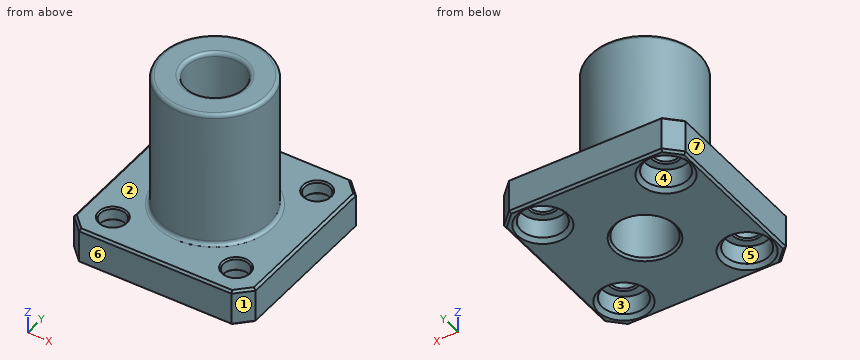
from build123d import *

# Parameters (mm, degrees)
SKETCH1_W                               = 25
SKETCH1_H                               = 25
SKETCH1_R                               = 4
BOSS_EXTRUDE1_DEPTH                     = 5
SKETCH2_R                               = 7.5
SKETCH2_R_2                             = 4
BOSS_EXTRUDE2_DEPTH                     = 19
CHAMFER1_SIZE                           = 2
CBORE_FOR_M3_PAN_HEAD_SCREW1_AT_2_COUNT = 2
CBORE_FOR_M3_PAN_HEAD_SCREW1_AT_2_PITCH = 16.970562748
CBORE_FOR_M3_PAN_HEAD_SCREW1_AT_3_COUNT = 2
CBORE_FOR_M3_PAN_HEAD_SCREW1_AT_3_PITCH = 24
CBORE_FOR_M3_PAN_HEAD_SCREW1_AT_4_COUNT = 2
CBORE_FOR_M3_PAN_HEAD_SCREW1_AT_4_PITCH = 16.970562748
CHAMFER2_SIZE                           = 0.3
FILLET1_R                               = 0.5
FILLET2_R                               = 0.5
CHAMFER3_SIZE                           = 0.3
FILLET3_R                               = 0.5
CHAMFER4_SIZE                           = 0.2


with BuildPart() as part:
    # Sketch1 → Boss-Extrude1 (new body)
    with BuildSketch(Plane.XY):
        Rectangle(SKETCH1_W, SKETCH1_H)
        Circle(SKETCH1_R, mode=Mode.SUBTRACT)
    extrude(amount=BOSS_EXTRUDE1_DEPTH)

    # Sketch2 → Boss-Extrude2 (add)
    with BuildSketch(Plane.XY.offset(5)):
        Circle(SKETCH2_R)
        Circle(SKETCH2_R_2, mode=Mode.SUBTRACT)
    extrude(amount=BOSS_EXTRUDE2_DEPTH)

    # Chamfer1
    chamfer1_edges = [part.edges().sort_by_distance(p)[0] for p in [
        (12.5, -12.5, 2.5),
        (-12.5, -12.5, 2.5),
        (-12.5, 12.5, 2.5),
        (12.5, 12.5, 2.5),
    ]]
    chamfer(chamfer1_edges, length=CHAMFER1_SIZE)

    # Sketch4 → CBORE for M3 Pan Head Screw1 (revolve, cut)
    with BuildSketch(Plane(origin=(8.485281374, 8.485281374, 0), x_dir=(0, 1, 0), z_dir=(1, 0, 0))):
        Polygon((0, 0), (0, 24), (1.75, 24), (1.75, 3.1), (3, 3.1), (3, 0.525), (3.525, 0), align=None)
    cbore_for_m3_pan_head_screw1 = revolve(axis=Axis((8.485281374, 8.485281374, -6.35), (0, 0, 1)), mode=Mode.SUBTRACT)

    # CBORE for M3 Pan Head Screw1 at 2: CBORE for M3 Pan Head Screw1 ×2
    with Locations(*[(-i * CBORE_FOR_M3_PAN_HEAD_SCREW1_AT_2_PITCH, 0, 0) for i in range(1, CBORE_FOR_M3_PAN_HEAD_SCREW1_AT_2_COUNT)]):
        add(cbore_for_m3_pan_head_screw1, mode=Mode.SUBTRACT)

    # CBORE for M3 Pan Head Screw1 at 3: CBORE for M3 Pan Head Screw1 ×2
    with Locations(*[Vector(-0.7071067811865676, -0.7071067811865276, 0) * (i * CBORE_FOR_M3_PAN_HEAD_SCREW1_AT_3_PITCH) for i in range(1, CBORE_FOR_M3_PAN_HEAD_SCREW1_AT_3_COUNT)]):
        add(cbore_for_m3_pan_head_screw1, mode=Mode.SUBTRACT)

    # CBORE for M3 Pan Head Screw1 at 4: CBORE for M3 Pan Head Screw1 ×2
    with Locations(*[(0, -i * CBORE_FOR_M3_PAN_HEAD_SCREW1_AT_4_PITCH, 0) for i in range(1, CBORE_FOR_M3_PAN_HEAD_SCREW1_AT_4_COUNT)]):
        add(cbore_for_m3_pan_head_screw1, mode=Mode.SUBTRACT)

    # Chamfer2
    chamfer2_edges = [part.edges().sort_by_distance(p)[0] for p in [
        (-12.5, 0, 0),
        (-12.5, 0, 5),
        (12.5, 0, 0),
        (0, -12.5, 0),
        (0, 12.5, 0),
        (11.5, 11.5, 0),
        (11.5, -11.5, 0),
        (-11.5, -11.5, 0),
        (-11.5, 11.5, 0),
        (0, 12.5, 5),
        (12.5, 0, 5),
        (0, -12.5, 5),
        (11.5, 11.5, 5),
        (11.5, -11.5, 5),
        (-11.5, -11.5, 5),
        (-11.5, 11.5, 5),
    ]]
    chamfer(chamfer2_edges, length=CHAMFER2_SIZE)

    # Fillet1
    fillet1_edges = [part.edges().sort_by_distance(p)[0] for p in [
        (-7.5, 0, 24),
    ]]
    fillet(fillet1_edges, radius=FILLET1_R)

    # Fillet2
    fillet2_edges = [part.edges().sort_by_distance(p)[0] for p in [
        (-4, 0, 24),
    ]]
    fillet(fillet2_edges, radius=FILLET2_R)

    # Chamfer3
    chamfer3_edges = [part.edges().sort_by_distance(p)[0] for p in [
        (-4, 0, 0),
    ]]
    chamfer(chamfer3_edges, length=CHAMFER3_SIZE)

    # Fillet3
    fillet3_edges = [part.edges().sort_by_distance(p)[0] for p in [
        (-7.5, 0, 5),
    ]]
    fillet(fillet3_edges, radius=FILLET3_R)

    # Chamfer4
    chamfer4_edges = [part.edges().sort_by_distance(p)[0] for p in [
        (8.485281374, -10.235281374, 5),
        (8.485281374, -10.235281374, 3.1),
        (-8.485281374, -10.235281374, 5),
        (-8.485281374, -10.235281374, 3.1),
        (-8.485281374, 6.735281374, 5),
        (-8.485281374, 6.735281374, 3.1),
        (8.485281374, 6.735281374, 5),
        (8.485281374, 6.735281374, 3.1),
    ]]
    chamfer(chamfer4_edges, length=CHAMFER4_SIZE)


solid = part.part
Part model, mm, in its own coordinate system. Face numbers are marked on the shaded views. A direction names the side the tool comes from. Coordinates: 2 decimals unless noted, no trailing zeros. Write each loop counter-clockwise with the first axis right and the second up, starting at its lowest first coordinate (ties: lowest second). Pieces come first, ordered by that corner, then holes. Notation, with made-up numbers: (8.5, 25) - (43.5, 25) arc R31 ccw to (43.5, 58) - close; hole circle Ø9 at (57.25, -24.75). An arc over 180 degrees is marked (long way). Put each result on its own line as item: value.
1. 3-axis set-ups, long thin cutter, end or side, ignore diameter. For the marked faces 1, 2 and 3: which of +Z, -Z, +X, -X, +Y, -Y reach the whole face in a straight line?
Final values:
face 1: +Z, -Z, +X, -Y
face 2: +Z
face 3: -Z
2. Band-saw the part on A-A (y = 0). Write the cut outline in (x, z).
Final values:
outline: (-12.5, 0.3) - (-12.2, 0) - (-4.3, 0) - (-4, 0.3) - (-4, 23.5) arc R0.5 ccw to (-4.5, 24) - (-7, 24) arc R0.5 ccw to (-7.5, 23.5) - (-7.5, 5.5) arc R0.5 cw to (-8, 5) - (-12.2, 5) - (-12.5, 4.7) - close; (4, 0.3) - (4.3, 0) - (12.2, 0) - (12.5, 0.3) - (12.5, 4.7) - (12.2, 5) - (8, 5) arc R0.5 cw to (7.5, 5.5) - (7.5, 23.5) arc R0.5 ccw to (7, 24) - (4.5, 24) arc R0.5 ccw to (4, 23.5) - close
3. Flat gauge pins, fed straight in: pin 1 Ø12 at (y, z) = (-3.5, 8) entering from -X; pin 2 Ø12 at (x, z) = (-0.5, 14) entering from +Y; pin 3 Ø5 at (x, z) = (3.5, 16) entering from +Y; pin 4 Ø5.5 at (x, y) = (8.49, 8.49) entering from -Z. Where does each tip first touch, or does it go through?
Final values:
pin 1: stops at x = -12.5
pin 2: stops at y = 7.5
pin 3: stops at y = 7.43
pin 4: stops at z = 3.1
4. Probe line 1 along Y through (x, z) = (0.25, 2); line 2 along Y through (x, z) = (0, 6); line 3 along Y through (x, z) = (11.25, 1.75). List the from-to ranges inside material, lowest first. Write a range as [from, to].
Final values:
line 1: y = [-12.5, -3.99], [3.99, 12.5]
line 2: y = [-7.5, -4], [4, 7.5]
line 3: y = [-11.75, -9.65], [-7.32, 7.32], [9.65, 11.75]
5. Band-saw the part on D-D (z = 13.25). Write the cut outline in (x, y).
Final values:
outline: circle Ø15 at (0, 0); hole circle Ø8 at (0, 0)
6. Band-saw the part on C-C (z = 4.25). Write the cut outline in (x, y).
Final values:
outline: (-12.5, -10.5) - (-10.5, -12.5) - (10.5, -12.5) - (12.5, -10.5) - (12.5, 10.5) - (10.5, 12.5) - (-10.5, 12.5) - (-12.5, 10.5) - close; hole circle Ø3.5 at (-8.49, -8.49); hole circle Ø3.5 at (-8.49, 8.49); hole circle Ø8 at (0, 0); hole circle Ø3.5 at (8.49, -8.49); hole circle Ø3.5 at (8.49, 8.49)
7. Two-plate mould, pull along Y, no slides. Class the marked faces 4, 5, 6 and 7: +Y half, -Y half, draft (parallel to the pull), parting line (faces both ways), or undercut.
Final values:
face 4: undercut
face 5: undercut
face 6: -Y half
face 7: draft
